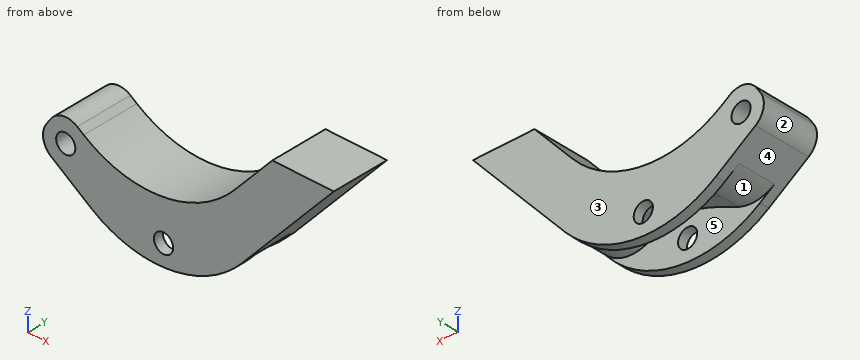
```python
from build123d import *

# Parameters (mm, degrees)
SKETCH3_R           = 2.5
BOSS_EXTRUDE2_DEPTH = 7.5
CUT_EXTRUDE2_DEPTH  = 5
FILLET1_START       = -5
FILLET1_DEPTH       = 10
FILLET2_R           = 5


with BuildPart() as part:
    # Sketch3 → Boss-Extrude2 (new, symmetric)
    with BuildSketch(Plane(origin=(0, 0, 0), x_dir=(1, 0, 0), z_dir=(0, 1, 0))):
        with BuildLine():
            Line((0, 0), (16.055459438, 0))
            Line((16.055459438, 0), (-7.935861068, 26.99023557))
            ThreePointArc((-7.935861068, 26.99023557), (-26.707018244, 36.836313291), (-47.300903293, 31.817001905))
            Line((-47.300903293, 31.817001905), (-61.838574124, 21.868238869))
            Line((-61.838574124, 21.868238869), (-55.061469058, 11.965166269))
            Line((-55.061469058, 11.965166269), (-49.247161684, 15.944150727))
            ThreePointArc((-49.247161684, 15.944150727), (-28.653276634, 20.963462112), (-9.882119459, 11.117384391))
            Line((-9.882119459, 11.117384391), (0, 0))
        make_face()
        with Locations(Location((-53.944540562, 20, 0), (0, 0, 270))):
            Circle(SKETCH3_R, mode=Mode.SUBTRACT)
        with Locations(Location((-28.408134096, 31.487077096, 0), (0, 0, 270))):
            Circle(SKETCH3_R, mode=Mode.SUBTRACT)
    extrude(amount=BOSS_EXTRUDE2_DEPTH, both=True)

    # Sketch6 → Cut-Extrude2 (cut, symmetric)
    with BuildSketch(Plane(origin=(0, 0, 0), x_dir=(1, 0, 0), z_dir=(0, 1, 0))):
        with BuildLine():
            add(Edge.make_bspline(
                [(-14.79224673, 32.705040265), (-17.331871812, 26.215966366), (-31.296858097, 23.259335294), (-41.248027481, 30.965132279), (-47.300903293, 31.817001905)],
                knots=[0, 0, 0, 0, 0.502708052, 1, 1, 1, 1], degree=3))
            ThreePointArc((-14.79224673, 32.705040265), (-31.177344469, 37.048133404), (-47.300903293, 31.817001905))
        make_face()
    extrude(amount=CUT_EXTRUDE2_DEPTH, both=True, mode=Mode.SUBTRACT)

    # Fillet1: read off the stored shape, not the designer's step
    # Fillet1 outline → Fillet1 (cut)
    with BuildSketch(Plane(origin=(0, 0, 0), x_dir=(1, 0, 0), z_dir=(0, 1, 0)).offset(FILLET1_START)):
        with BuildLine():
            ThreePointArc((-19.221952817, 27.410351809), (-12.561308079, 28.72495355), (-6.596181971, 25.483096586))
            Line((-6.596181971, 25.483096586), (-7.935861068, 26.99023557))
            ThreePointArc((-7.935861068, 26.99023557), (-11.150327664, 30.10405779), (-14.79224673, 32.705040265))
            add(Edge.make_bspline(
                [(-14.79224673, 32.705040265), (-15.739998483, 30.283410709), (-17.311764452, 28.558502186), (-19.221952817, 27.410351809)],
                knots=[0, 0, 0, 0, 0.187603454, 0.187603454, 0.187603454, 0.187603454], degree=3))
        make_face()
        with BuildLine():
            ThreePointArc((-51.091167548, 29.223158548), (-46.575226496, 30.906360534), (-41.796439127, 30.281793648))
            add(Edge.make_bspline(
                [(-41.796439127, 30.281793648), (-43.564588599, 30.974367456), (-45.376964166, 31.546230564), (-47.300903293, 31.817001905)],
                knots=[0.84193308, 0.84193308, 0.84193308, 0.84193308, 1, 1, 1, 1], degree=3))
            Line((-47.300903293, 31.817001905), (-51.091167548, 29.223158548))
        make_face()
    extrude(amount=FILLET1_DEPTH, mode=Mode.SUBTRACT)

    # Fillet2
    fillet2_edges = [part.edges().sort_by_distance(p)[0] for p in [
        (-55.061469058, 0, -11.965166269),
        (-61.838574124, 0, -21.868238869),
    ]]
    fillet(fillet2_edges, radius=FILLET2_R)


solid = part.part
```
Can you work these out from the model? Positions are in its coordinate system, mm. Face numbers are marked on the shaded views. A direction names the side the tool comes from. Coordinates: 2 decimals unless noted, no trailing zeros. Loops run counter-clockwise (first coordinate to the right, second up) from the corner with the lowest first, then second, coordinate; pieces in that order, holes last. Notation, with made-up numbers: M 12.5,-14.75 L 54.5,-14.75 A18 ccw 54.5,20.25 Z; hole C 57,53.25 d8. An arc over 180 degrees is marked long. Put each result on its own line as item: value. Start each with the question number.
(1) Imagine slicing it at A-A on y = -6.5. List the corners of the cut face in (x, z) for me, and give its area (3 significant figures).
(2) Imagine slicing it at B-B on z = -20. List the corners of the cut face in (x, y) for me, and give its area (3 significant figures).
(3) Will these pins go through, and if not, where does the flat tip stop? pin 1 Ø6 at (y, z) = (5.5, -8) entering from +X; pin 2 Ø3 at (x, z) = (-53.94, -20) entering from -Y; pin 3 Ø1.5 at (y, z) = (-2, -16) entering from +X; pin 4 Ø1 at (x, y) = (-51, -5) entering from -Z.
(4) Imagine slicing it at D-D on x = -27. Give the number of separate pieces and of enclosed holes in the cut face, and give its area (3 significant figures).
(5) I need wall thicknesses on probe 1 along Y at (x, z) = (-33.5, -32); probe 2 along X at (y, z) = (-6.5, -31); probe 3 along X at (y, z) = (-1.5, -7). Which ranges of each line are inside material? Lowest first, please.
(6) Imagine slicing it at C-C on x = -48.5. List the corners of the cut face in (y, z) for me, and give its area (3 significant figures).
(7) We'd pull the mould along Y, two halves only. Please class the marked faces 3, 4 and 5: +Y half, -Y half, draft (parallel to the pull), parting line (faces both ways), or undercut.
(8) Which directions (+Z, -Z, +X, -X, +Y, -Y) give clear straight access to the entire face, cutting with the end or side of a thin tool? Please do the marked faces 1 and 2.
Worked answers:
1. outline: M -59.01,-17.74 A5 ccw -57.71,-24.69 L -47.3,-31.82 A30 ccw -7.94,-26.99 L 16.06,0 L 0,0 L -9.88,-11.12 A30 cw -49.25,-15.94 L -50.94,-14.79 A5 ccw -57.89,-16.09 Z; hole C -53.94,-20 d5; hole C -28.41,-31.49 d5
1. area: 1,040 mm2
2. outline: M -59.86,-7.5 L -56.44,-7.5 L -56.44,7.5 L -59.86,7.5 Z; M -51.44,-7.5 L -40.66,-7.5 L -40.66,7.5 L -51.44,7.5 Z; M -23.95,-7.5 L -1.72,-7.5 L -1.72,7.5 L -23.95,7.5 Z
2. area: 546 mm2
3. pin 1: stops at x = 11.61
3. pin 2: passes through
3. pin 3: stops at x = 2.5
3. pin 4: stops at z = -29.63
4. separate pieces: 3
4. enclosed holes: 0
4. area: 109 mm2
5. probe 1: y = -7.5 to -5, 5 to 7.5
5. probe 2: x = -48.49 to -30.86, -25.96 to -12.28
5. probe 3: x = -6.22 to 9.83
6. outline: M -7.5,-31 L -5,-31 L -5,-30.49 L 5,-30.49 L 5,-31 L 7.5,-31 L 7.5,-16.44 L -7.5,-16.44 Z
6. area: 213 mm2
7. face 3: +Y half
7. face 4: draft
7. face 5: undercut
8. face 1: -Z
8. face 2: -X, +Y, -Y
